Autodesk Inventor part; units mm, degrees
ref_plane "YZ Plane" through (0, 0, 0) normal (1, 0, 0) x (0, 1, 0)
ref_plane "XZ Plane" through (0, 0, 0) normal (0, 1, 0) x (-1, 0, 0)
ref_plane "XY Plane" through (0, 0, 0) normal (0, 0, 1) x (1, 0, 0)
sketch "Skizze1" plane through (0, 0, 0) normal (0, 1, 0) x (-1, 0, 0)
  line L0 (-1.8, 15) -> (8.2, 15)
  line L1 (8.2, 15) -> (8.2, -15)
  line L2 (8.2, -15) -> (-1.8, -15)
  line L3 (16.5068, 0) -> (-47.7946, 0) construction
  arc A0 (-9.3, 7.5) -> (-9.3, -7.5) centre (-9.3, 0) ccw
  circle A1 centre (-9.3, 0) radius 5.15
  line L4 (-1.8, -15) -> (-1.8, -7.5)
  line L5 (-1.8, 7.5) -> (-1.8, 15)
  line L6 (-9.3, 7.5) -> (-1.8, 7.5)
  line L7 (-9.3, -7.5) -> (-1.8, -7.5)
  point P0 (0, 0)
  dimension "d0" = 30
  dimension "d1" = 15
  dimension "d2" = 10.3
  dimension "d3" = 15
  dimension "d7" = 10
  dimension "d8" = 17.5
  dimension "d14" = 7.5
  dimension "d15" = 7.5
  dimension "d16" = 1.8
  dimension "d17" = 1.8
extrude "Extrusion1" add sketch "Skizze1" along normal blind 10
properties part number "Achsenhalterung"
The listing builds one solid part. Answer for the finished solid, in the listing's coordinates (mm). A direction names the side the tool comes from. Round coordinates to 2 decimals unless told otherwise and drop trailing zeros. Write each loop counter-clockwise with the first axis right and the second up, starting at its lowest first coordinate (ties: lowest second). Pieces come first, ordered by that corner, then holes. Notation, with made-up numbers: (-8, -10.75) - (35, -10.75) arc R12 ccw to (35, -0.75) - close; hole circle Ø5 at (-33, 70). An arc over 180 degrees is marked (long way). Use one line per item in the form item = value. Start each with the question number.
Item 1: A cutting plane is placed at D-D (z = 13.25). Write down the section's boundary in (x, y).
Item 2: A tool of negligible diameter and unlimited length cuts with its end or side. For faces 1 (the flat face through (6, 5, -7.5)), 2 (the flat face through (-3, 5, -15)), from which of +Z, -Z, +X, -X, +Y, -Y can it reach the whole face along a straight path? Write none if from no direction.
Item 3: Determine the mould class of faces 3 (the flat face through (1.8, 5, 11)), 4 (the flat face through (6, 5, 7.5)), 5 (the cylindrical face through (14.445, 4.93, -0.226)) for opening direction Z: +Z half, -Z half, draft (parallel to the pull), parting line (faces both ways), or undercut.
Item 4: A cutting plane is placed at B-B (x = 7.75). Write down the section's boundary in (y, z), plus the area to 3 significant figures.
Item 5: Flat-ended cylindrical pins translate along their axes: pin 1 Ø2 at (x, y) = (3, 5) entering from -Z; pin 2 Ø6 at (y, z) = (2.5, -12) entering from +X; pin 3 Ø4 at (x, y) = (4.5, 3.5) entering from +Z. Find the tip coordinate at first contact, or state that the pin passes through.
Item 6: A cutting plane is placed at C-C (y = 7.5). Write down the section's boundary in (x, z).
Item 7: Find the intervals of material crossed by line 1 (Z direction, x = 9.3, y = 2.5); line 2 (X direction, y = 7.75, z = 9.5); line 3 (Z direction, x = 5.25, y = 6.25), in increasing order. Write a range as [from, to].
Item 8: A cutting plane is placed at A-A (z = 0). Write down the section's boundary in (x, y), plus the area to 3 significant figures.
The answers:
q1.outline = (-8.2, 0) - (1.8, 0) - (1.8, 10) - (-8.2, 10) - close
q2.face_1 = -Z, +X, +Y, -Y
q2.face_2 = -Z, +X, -X, +Y, -Y
q3.face_3 = draft
q3.face_4 = +Z half
q3.face_5 = undercut
q4.outline = (0, -7.5) - (10, -7.5) - (10, -4.91) - (0, -4.91) - close; (0, 4.91) - (10, 4.91) - (10, 7.5) - (0, 7.5) - close
q4.area = 51.8 mm^2
q5.pin_1 = -7.5
q5.pin_2 = 1.8
q5.pin_3 = 7.5
q6.outline = (-8.2, -15) - (1.8, -15) - (1.8, -7.5) - (9.3, -7.5) arc R7.5 ccw to (9.3, 7.5) - (1.8, 7.5) - (1.8, 15) - (-8.2, 15) - close; hole circle Ø10.3 at (9.3, 0)
q7.line_1 = [-7.5, -5.15], [5.15, 7.5]
q7.line_2 = [-8.2, 1.8]
q7.line_3 = [-7.5, -3.18], [3.18, 7.5]
q8.outline = (-8.2, 0) - (4.15, 0) - (4.15, 10) - (-8.2, 10) - close; (14.45, 0) - (16.8, 0) - (16.8, 10) - (14.45, 10) - close
q8.area = 147 mm^2
